from build123d import *

# Parameters (mm, degrees)
SKETCH_1_R          = 6
EXTRUDE_1_DEPTH     = 120
CUT_EXTRUDE_START   = -3.5
CUT_EXTRUDE_1_DEPTH = 10
SKETCH_3_W          = 1.1
SKETCH_3_H          = 0.5
CHAMFER_1_SIZE      = 0.5


with BuildPart() as part:
    # 草图1 → 凸台-拉伸1 (new body)
    with BuildSketch(Plane.XY):
        Circle(SKETCH_1_R)
    extrude(amount=EXTRUDE_1_DEPTH)

    # 草图2 → 切除-拉伸1 (cut)
    with BuildSketch(Plane(origin=(0, 0, 0), x_dir=(1, 0, 0), z_dir=(0, 1, 0)).offset(CUT_EXTRUDE_START)):
        with BuildLine():
            Line((2, -58), (2, -84))
            ThreePointArc((2, -84), (0, -86), (-2, -84))
            Line((-2, -84), (-2, -58))
            ThreePointArc((-2, -58), (0, -56), (2, -58))
        make_face()
    extrude(amount=-CUT_EXTRUDE_1_DEPTH, mode=Mode.SUBTRACT)

    # 草图3 → 切除-旋转1 (revolve, cut)
    with BuildSketch(Plane(origin=(0, 0, 0), x_dir=(0, 0, -1), z_dir=(1, 0, 0)), mode=Mode.PRIVATE) as cut_revolve_1_sk:
        with Locations((-88.05, 5.75)):
            Rectangle(SKETCH_3_W, SKETCH_3_H)
        with Locations((-34.55, 5.75)):
            Rectangle(SKETCH_3_W, SKETCH_3_H)
        with Locations((-52.95, 5.75)):
            Rectangle(SKETCH_3_W, SKETCH_3_H)
    revolve(cut_revolve_1_sk.sketch.rotate(Axis((0, 0, 130.661115057), (0, 0, -1)), 90), axis=Axis((0, 0, 130.661115057), (0, 0, -1)), mode=Mode.SUBTRACT)

    # 倒角1
    chamfer_1_edges = [part.edges().sort_by_distance(p)[0] for p in [
        (-6, 0, 0),
        (-6, 0, 120),
    ]]
    chamfer(chamfer_1_edges, length=CHAMFER_1_SIZE)


solid = part.part
The listing builds one solid part. Answer for the finished solid, in the listing's coordinates (mm). A direction names the side the tool comes from. Coordinates: 2 decimals unless noted, no trailing zeros. Order: outer loops, then holes, each group sorted by start corner. A loop starts at its lowest first (then second) coordinate and runs counter-clockwise, first axis right, second up.
Q1. Consider line 1 (Z direction, x = -4.75, y = 3); line 2 (Y direction, x = 0.5, z = 30.5); line 3 (X direction, y = -4.75, z = 78). Determine where each line is inside the solid, lowest interval first.
Q2. A cutting plane is placed at A-A, the plane z = 24. Write down the section's boundary in (x, y), and give its area (3 significant figures).
Q3. Given P1, Ø1, axis at x = -4, z = 49, coming from the -Y side; P2, Ø1.7, axis at y = -4.5, z = 75, coming from the -X side; P3, Ø3.5, axis at x = 0, y = 0.5, coming from the -Z side; P4, Ø3, axis at x = -4, z = 54.5, coming from the +Y side, each flat-ended and moving along its own axis, determine where each tip first touches the part or whether it passes through.
Q4. Which of the six approach directions +Z, -Z, +X, -X, +Y, -Y give full straight-line access (tool end or side, diameter ignored) to faces 1 (the face through (-6, 0, 104)), 2 (the face through (0, -3.5, 71)), 3 (the face through (-3, 5, 52.4))?
Q5. For a pull along X with two mould halves and no side action, classify faces 4 (the face through (0, -5, 56)), 5 (the face through (-3, 5, 88.6)), 6 (the face through (-1.19, 5.37, 34.54)) as pulls with the +X half, pulls with the -X half, needs draft (parallel to the pull), parting line crosses it, or undercut.
Answers follow:
1. line 1: z = 0.12 to 34, 35.1 to 52.4, 53.5 to 87.5, 88.6 to 119.88
1. line 2: y = -5.98 to 5.98
1. line 3: x = -3.67 to -2, 2 to 3.67
2. outline: circle Ø12 at (0, 0)
2. area: 113 mm2
3. P1: stops at y = -4.87
3. P2: stops at x = -4.76
3. P3: stops at z = 0
3. P4: stops at y = 5.45
4. face 1: +Z, -Z
4. face 2: -Y
4. face 3: none
5. face 4: undercut
5. face 5: needs draft
5. face 6: parting line crosses it
